Model file for the job. Use its own axes, mm. Face numbers are marked on the shaded views. A direction names the side the tool comes from. Coordinates: 2 decimals unless noted, no trailing zeros. Write each loop counter-clockwise with the first axis right and the second up, starting at its lowest first coordinate (ties: lowest second). Pieces come first, ordered by that corner, then holes. Notation, with made-up numbers: M -10.5,13 L -0.5,13 A24 cw -0.5,50 Z; hole C -29,-2 d7. An arc over 180 degrees is marked long. Answer in a Markdown table with one row per item. Add a question column.
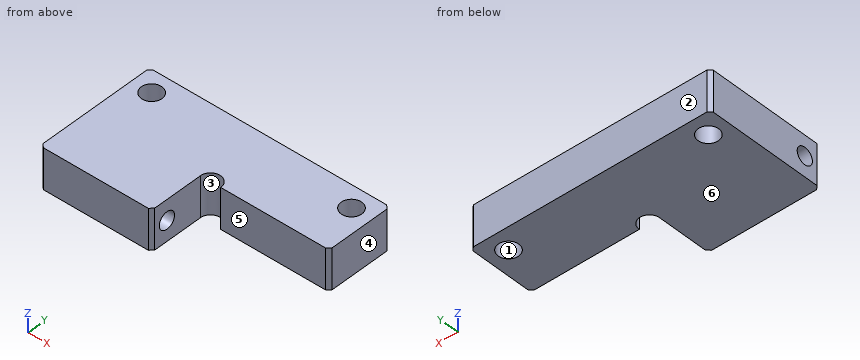
```python
from build123d import *

# Parameters (mm, degrees)
SKETCH_1_W          = 35.6
SKETCH_1_H          = 18
EXTRUDE_1_DEPTH     = 6
SKETCH_3_W          = 2.5
SKETCH_3_H          = 16
CUT_EXTRUDE_1_DEPTH = 28
SKETCH_4_W          = 16.55
SKETCH_4_H          = 8
CUT_EXTRUDE_2_DEPTH = 10
HOLE_WIZARD_M3_1_D  = 2.5
SKETCH_8_R          = 1.525
CUT_EXTRUDE_3_DEPTH = 22
CHAMFER_1_SIZE      = 0.5
SKETCH_9_R          = 1.5
CUT_EXTRUDE_4_DEPTH = 10


with BuildPart() as part:
    # 草图1 → 凸台-拉伸1 (new body)
    with BuildSketch(Plane.XY):
        Rectangle(SKETCH_1_W, SKETCH_1_H)
    extrude(amount=EXTRUDE_1_DEPTH)

    # 草图3 → 切除-拉伸1 (cut)
    with BuildSketch(Plane(origin=(0, 0, 0), x_dir=(-1, 0, 0), z_dir=(0, 0, -1))):
        with Locations((0, -9)):
            Rectangle(SKETCH_3_W, SKETCH_3_H)
    extrude(amount=-CUT_EXTRUDE_1_DEPTH, mode=Mode.SUBTRACT)

    # 草图4 → 切除-拉伸2 (cut)
    with BuildSketch(Plane(origin=(0, 0, 0), x_dir=(-1, 0, 0), z_dir=(0, 0, -1))):
        with Locations((-9.525, -5)):
            Rectangle(SKETCH_4_W, SKETCH_4_H)
    extrude(amount=-CUT_EXTRUDE_2_DEPTH, mode=Mode.SUBTRACT)

    # M3 螺纹孔1 (through all)
    with Locations(Plane(origin=(-1.25, 0, 0), x_dir=(0, 0, -1), z_dir=(1, 0, 0))):
        with Locations((-3, -6.5)):
            Hole(HOLE_WIZARD_M3_1_D / 2)

    # 草图8 → 切除-拉伸3 (cut)
    with BuildSketch(Plane.XY.offset(6)):
        with Locations((-14.8, 6)):
            Circle(SKETCH_8_R)
        with Locations(Location((14.8, 6, 0), (0, 0, 180))):
            Circle(SKETCH_8_R)
    extrude(amount=-CUT_EXTRUDE_3_DEPTH, mode=Mode.SUBTRACT)

    # 倒角1
    chamfer_1_edges = [part.edges().sort_by_distance(p)[0] for p in [
        (-1.25, -9, 3),
        (17.8, -1, 3),
        (-17.8, -9, 3),
        (-17.8, 9, 3),
        (17.8, 9, 3),
    ]]
    chamfer(chamfer_1_edges, length=CHAMFER_1_SIZE)

    # 草图9 → 切除-拉伸4 (cut)
    with BuildSketch(Plane.XY.offset(6)):
        with Locations((0.25, -1)):
            Circle(SKETCH_9_R)
    extrude(amount=-CUT_EXTRUDE_4_DEPTH, mode=Mode.SUBTRACT)


solid = part.part
```
1) Drill centre lines: probe 1 along X at (y, z) = (7, 2.75); probe 2 along X at (y, z) = (6.5, 3.2); probe 3 along Y at (x, z) = (-2, 3.05). Where is each one in solid material? Low to high.
2) Slice it at A-A (x = -14.8). Give the cut face in (y, z) (3 decimals), then the cut area to 3 significant figures.
3) Slice it at D-D (z = 1). Give the cut face in (x, y) (3 decimals), then the cut area to 3 significant figures.
4) Slice it at C-C (y = -6.5). Give the cut face in (x, z), then the cut area to 3 significant figures.
5) Two-plate mould, pull along X, no slides. Class the marked faces 1, 2, 3 and 4: released by +X, released by -X, zero draft, split by the parting line, or undercut.
6) Which spindle directions (+Z, -Z, +X, -X, +Y, -Y) get a long thin tool onto all of the face, cutting with end or side? Do the marked faces 5 and 6. Say none if no direction does.
7) Flat gauge pin, fed straight in: pin 1 Ø2.5 at (x, y) = (14.8, 6) entering from +Z. Where does the tip first touch, or does it go through?
8) Slice it at B-B (z = 3). Give the cut face in (x, y) (3 decimals), then the cut area to 3 significant figures.
Ans:
| question | item | result |
|---|---|---|
| 1 | probe 1 | x = -17.8 to -15.95, -13.65 to 13.65, 15.95 to 17.8 |
| 1 | probe 2 | x = -17.8 to -16.24, -13.36 to 13.36, 16.24 to 17.8 |
| 1 | probe 3 | y = -9 to -7.75, -5.25 to 9 |
| 2 | outline | M -9,0 L 4.475,0 L 4.475,6 L -9,6 Z; M 7.525,0 L 9,0 L 9,6 L 7.525,6 Z; hole C -6.5,3 d2.5 |
| 2 | area | 84.8 mm2 |
| 3 | outline | M -17.8,-8.5 L -17.3,-9 L -1.75,-9 L -1.25,-8.5 L -1.25,-1 A1.5 cw 1.75,-1 L 17.3,-1 L 17.8,-0.5 L 17.8,8.5 L 17.3,9 L -17.3,9 L -17.8,8.5 Z; hole C -14.8,6 d3.05; hole C 14.8,6 d3.05 |
| 3 | area | 470 mm2 |
| 4 | outline | M -17.8,0 L -1.25,0 L -1.25,1.75 L -17.8,1.75 Z; M -17.8,4.25 L -1.25,4.25 L -1.25,6 L -17.8,6 Z |
| 4 | area | 57.9 mm2 |
| 5 | face 1 | undercut |
| 5 | face 2 | zero draft |
| 5 | face 3 | undercut |
| 5 | face 4 | released by +X |
| 6 | face 5 | +Z, -Z, +X, -Y |
| 6 | face 6 | -Z, +X, -X, +Y, -Y |
| 7 | pin 1 | passes through |
| 8 | outline | M -17.8,-8.5 L -17.3,-9 L -1.75,-9 L -1.25,-8.5 L -1.25,-7.75 L -17.8,-7.75 Z; M -17.8,-5.25 L -1.25,-5.25 L -1.25,-1 A1.5 cw 1.75,-1 L 17.3,-1 L 17.8,-0.5 L 17.8,8.5 L 17.3,9 L -17.3,9 L -17.8,8.5 Z; hole C -14.8,6 d3.05; hole C 14.8,6 d3.05 |
| 8 | area | 428 mm2 |
